from build123d import *

# Parameters (mm, degrees)
BOSS_EXTRUDE1_DEPTH = 1.5
BOSS_EXTRUDE2_DEPTH = 1.5
SKETCH3_W           = 0.5
SKETCH3_H           = 0.8
CUT_EXTRUDE1_DEPTH  = 400.124667241
SKETCH4_W           = 365.290263007
SKETCH4_H           = 79.626519776
BOSS_EXTRUDE3_DEPTH = 1.6
SKETCH5_W           = 14
SKETCH5_H           = 14
CUT_EXTRUDE2_DEPTH  = 400.133887311


with BuildPart() as part:
    # Sketch1 → Boss-Extrude1 (new body)
    with BuildSketch(Plane(origin=(0, 0, 0), x_dir=(1, 0, 0), z_dir=(0, 1, 0))):
        with BuildLine():
            Line((2, 0), (384, 0))
            ThreePointArc((384, 0), (385.414213562, 0.585786438), (386, 2))
            Line((386, 2), (386, 94))
            ThreePointArc((386, 94), (385.414213562, 95.414213562), (384, 96))
            Line((384, 96), (2, 96))
            ThreePointArc((2, 96), (0.585786438, 95.414213562), (0, 94))
            Line((0, 94), (0, 2))
            ThreePointArc((0, 2), (0.585786438, 0.585786438), (2, 0))
        make_face()
    extrude(amount=BOSS_EXTRUDE1_DEPTH)

    # Sketch2 → Boss-Extrude2 (add)
    with BuildSketch(Plane(origin=(0, 1.5, 0), x_dir=(1, 0, 0), z_dir=(0, 1, 0))):
        Polygon((343.8928, 96), (338, 101.5), (328, 101.5), (322.1072, 96), align=None)
    extrude(amount=-BOSS_EXTRUDE2_DEPTH)

    # Sketch3 → Cut-Extrude1 (cut, through all)
    with BuildSketch(Plane(origin=(0, 1.5, 0), x_dir=(1, 0, 0), z_dir=(0, 1, 0))):
        with Locations((328.57, 100.85)):
            Rectangle(SKETCH3_W, SKETCH3_H)
        with Locations((337.43, 100.85)):
            Rectangle(SKETCH3_W, SKETCH3_H)
    extrude(amount=-CUT_EXTRUDE1_DEPTH, mode=Mode.SUBTRACT)

    # Sketch4 → Boss-Extrude3 (add)
    with BuildSketch(Plane.XZ):
        with Locations((192.889995692, -46.221612613)):
            Rectangle(SKETCH4_W, SKETCH4_H)
    extrude(amount=BOSS_EXTRUDE3_DEPTH)

    # Sketch5 → Cut-Extrude2 (cut, through all)
    with BuildSketch(Plane(origin=(0, 1.5, 0), x_dir=(1, 0, 0), z_dir=(0, 1, 0))):
        with Locations((10, 86)):
            Rectangle(SKETCH5_W, SKETCH5_H)
    extrude(amount=-CUT_EXTRUDE2_DEPTH, mode=Mode.SUBTRACT)


solid = part.part
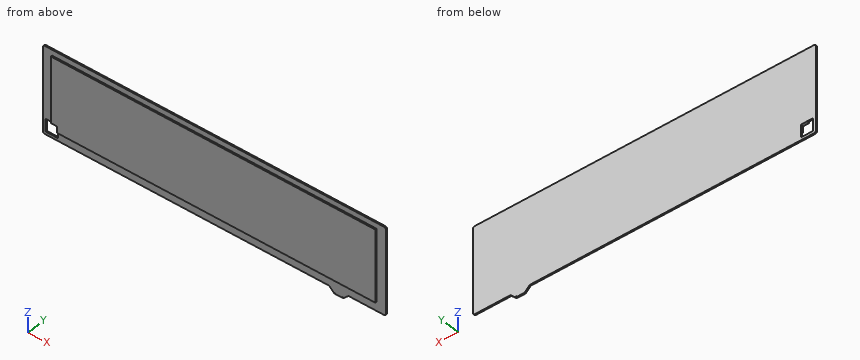
CAD build for the part. Positions are in the model's coordinates, mm. Coordinates: 2 decimals unless noted, no trailing zeros. Loops run counter-clockwise (first coordinate to the right, second up) from the corner with the lowest first, then second, coordinate; pieces in that order, holes last. Notation, with made-up numbers: (4, -29.5) - (17, -29.5) arc R25 cw to (17, 6.5) - close; hole circle Ø7 at (-34, -10). An arc over 180 degrees is marked (long way). Use one line per item in the form item = value. Start each with the question number.
1) Drill centre lines: L1, parallel to X at y = 0.8, z = -79.5; L2, parallel to X at y = -0.35, z = -59; L3, parallel to Z at x = 113, y = 0.6. Where is each one in solid material? Low to high. Write a range as from..to.
2) Flat gauge pins, fed straight in: pin 1 (1.8 mm diameter, centred on x = 268.5, y = -1, fed in from +Z); pin 2 (1.6 mm diameter, centred on x = 8.5, y = 0.5, fed in from -Z); pin 3 (1 mm diameter, centred on y = -1, z = -52.5, fed in from -X). Where does each tip first touch, or does it go through?
3) Band-saw the part on A-A (y = 0.8). Give the cut face in (x, z), and give its area (3 significant figures).
4) Band-saw the part on B-B (z = -24). Give the cut face in (x, y), and give its area (3 significant figures).
5) Band-saw the part on C-C (x = 157). Give the cut face in (y, z).
Check values:
q1.L1 = 0..3, 17..386
q1.L2 = 10.24..375.54
q1.L3 = -96..0
q2.pin_1 = -6.41
q2.pin_2 = -96
q2.pin_3 = 10.24
q3.outline = (0, -94) arc R2 ccw to (2, -96) - (322.11, -96) - (328, -101.5) - (338, -101.5) - (343.89, -96) - (384, -96) arc R2 ccw to (386, -94) - (386, -2) arc R2 ccw to (384, 0) - (2, 0) arc R2 ccw to (0, -2) - close; hole (3, -93) - (17, -93) - (17, -79) - (3, -79) - close; hole (328.32, -101.25) - (328.82, -101.25) - (328.82, -100.45) - (328.32, -100.45) - close; hole (337.18, -101.25) - (337.68, -101.25) - (337.68, -100.45) - (337.18, -100.45) - close
q3.area = 36,900 mm2
q4.outline = (0, 0) - (10.24, 0) - (10.24, -1.6) - (375.54, -1.6) - (375.54, 0) - (386, 0) - (386, 1.5) - (0, 1.5) - close
q4.area = 1,160 mm2
q5.outline = (-1.6, -86.03) - (0, -86.03) - (0, -96) - (1.5, -96) - (1.5, 0) - (0, 0) - (0, -6.41) - (-1.6, -6.41) - close
